The listing builds one solid part. Answer for the finished solid, in the listing's coordinates (mm). A direction names the side the tool comes from. Give positions to 0.01 mm unless a question says otherwise; leave off trailing zeros. Loops run counter-clockwise (first coordinate to the right, second up) from the corner with the lowest first, then second, coordinate; pieces in that order, holes last. Notation, with made-up numbers: (-39.75, 4.5) - (-28.75, 4.5) arc R24 cw to (-28.75, 38.5) - close; hole circle Ø6 at (73, 16.5). An arc over 180 degrees is marked (long way). Write item = value, one per line. Start each with the question number.
1) The part is cut by section B-B on y = 1.9. Write down the section's boundary in (x, z).
2) Consider probe 1 along Z at (x, y) = (-1.5, 1.4); probe 2 along X at (y, z) = (1, 0); probe 3 along Z at (x, y) = (0.5, 2.8). Determine where each line is inside the solid, lowest interval first.
3) Which of the six approach directions +Z, -Z, +X, -X, +Y, -Y give full straight-line access (tool end or side, diameter ignored) to faces 1 (the flat face through (-2, 0.4, -4.2)), 2 (the flat face through (-1.4, 0.3, -5.25)), 3 (the flat face through (2, 0.4, -4.2)), 4 (the flat face through (-1, 3, -1)), 5 (the flat face through (0, 2, -5.25))?
4) The mould has two halves that part along Z. Classify faces 6 (the cylindrical face through (0.345, 1.479, 1.097)), 7 (the flat face through (0, 0.816, -4)), 8 (the cylindrical face through (1.163, 0.397, -17.082)), 9 (the flat face through (1.5, 0.3, -5.25)): +Z half, -Z half, draft (parallel to the pull), parting line (faces both ways), or undercut.
5) Flat-ended cylindrical pins translate along their axes: P1, Ø2, axis at x = 2.5, z = -23, coming from the -Y side; P2, Ø3, axis at x = 0, z = 0, coming from the +Y side; P3, Ø2, axis at x = 3, z = -19, coming from the -Y side; P4, Ø1.5, axis at y = 0.5, z = -5, coming from the -X side. Find the tip coordinate at first contact, or state that the pin passes through.
6) The part is cut by section C-C on z = -22. Write down the section's boundary in (x, y).
7) The part is cut by section A-A on z = 0. Write down the section's boundary in (x, y).
from build123d import *

# Parameters (mm, degrees)
ESBO_O1_W                = 8
ESBO_O1_H                = 6.5
ESBO_O1_R                = 1.15
RESSALTO_EXTRUS_O1_DEPTH = 3
ESBO_O2_W                = 4
ESBO_O2_H                = 0.815950815
RESSALTO_EXTRUS_O2_DEPTH = 2
ESBO_O3_R                = 1.9
RESSALTO_EXTRUS_O3_DEPTH = 24


with BuildPart() as part:
    # Esboço1 → Ressalto-extrusão1 (new body)
    with BuildSketch(Plane(origin=(0, 0, 0), x_dir=(1, 0, 0), z_dir=(0, 1, 0))):
        Rectangle(ESBO_O1_W, ESBO_O1_H)
        with Locations(Location((0, 0, 0), (0, 0, 270))):
            Circle(ESBO_O1_R, mode=Mode.SUBTRACT)
    extrude(amount=RESSALTO_EXTRUS_O1_DEPTH)

    # Esboço2 → Ressalto-extrusão2 (add)
    with BuildSketch(Plane(origin=(0, 0, -3.25), x_dir=(-1, 0, 0), z_dir=(0, 0, -1))):
        with Locations((0, 0.407975407)):
            Rectangle(ESBO_O2_W, ESBO_O2_H)
    extrude(amount=RESSALTO_EXTRUS_O2_DEPTH)

    # Esboço3 → Ressalto-extrusão3 (add)
    with BuildSketch(Plane(origin=(0, 0, -5.25), x_dir=(-1, 0, 0), z_dir=(0, 0, -1))):
        with Locations(Location((0, 1.9, 0), (0, 0, 214.788741518))):
            Circle(ESBO_O3_R)
    extrude(amount=RESSALTO_EXTRUS_O3_DEPTH)


solid = part.part
Answer below:
q1.outline = (-4, -3.25) - (4, -3.25) - (4, 3.25) - (-4, 3.25) - close; (-1.9, -29.25) - (1.9, -29.25) - (1.9, -5.25) - (-1.9, -5.25) - close; hole circle Ø2.3 at (0, 0)
q2.probe_1 = -29.25 to -5.25, -3.25 to 3.25
q2.probe_2 = -4 to -1.15, 1.15 to 4
q2.probe_3 = -29.25 to -5.25, -3.25 to -1.04, 1.04 to 3.25
q3.face_1 = -Z, -X, +Y, -Y
q3.face_2 = -Z, -X, -Y
q3.face_3 = -Z, +X, +Y, -Y
q3.face_4 = +Z, +X, -X, +Y
q3.face_5 = +X, -X, +Y
q4.face_6 = undercut
q4.face_7 = undercut
q4.face_8 = draft
q4.face_9 = -Z half
q5.P1 = 0.73
q5.P2 = 3
q5.P3 = through
q5.P4 = -2
q6.outline = circle Ø3.8 at (0, 1.9)
q7.outline = (-4, 0) - (-1.15, 0) - (-1.15, 3) - (-4, 3) - close; (1.15, 0) - (4, 0) - (4, 3) - (1.15, 3) - close
